from build123d import *

# Parameters (mm, degrees)
SKETCH1_W           = 55
SKETCH1_H           = 28
BOSS_EXTRUDE1_DEPTH = 50
SKETCH2_R           = 14
BOSS_EXTRUDE2_DEPTH = 5
SKETCH3_R           = 3.5
BOSS_EXTRUDE3_DEPTH = 7
SKETCH4_W           = 11
SKETCH4_H           = 28
BOSS_EXTRUDE4_DEPTH = 3
CUT_EXTRUDE1_DEPTH  = 3


with BuildPart() as part:
    # Sketch1 → Boss-Extrude1 (new body)
    with BuildSketch(Plane(origin=(0, 0, 0), x_dir=(1, 0, 0), z_dir=(0, 1, 0))):
        Rectangle(SKETCH1_W, SKETCH1_H)
    extrude(amount=BOSS_EXTRUDE1_DEPTH)

    # Sketch2 → Boss-Extrude2 (add)
    with BuildSketch(Plane(origin=(0, 50, 0), x_dir=(1, 0, 0), z_dir=(0, 1, 0))):
        with Locations(Location((-13.5, 0, 0), (0, 0, 270))):
            Circle(SKETCH2_R)
    extrude(amount=BOSS_EXTRUDE2_DEPTH)

    # Sketch3 → Boss-Extrude3 (add)
    with BuildSketch(Plane(origin=(0, 55, 0), x_dir=(1, 0, 0), z_dir=(0, 1, 0))):
        with Locations(Location((-13.5, 0, 0), (0, 0, 270))):
            Circle(SKETCH3_R)
    extrude(amount=BOSS_EXTRUDE3_DEPTH)

    # Sketch4 → Boss-Extrude4 (add)
    with BuildSketch(Plane(origin=(0, 41.5, 0), x_dir=(1, 0, 0), z_dir=(0, 1, 0))):
        with Locations((33, 0)):
            Rectangle(SKETCH4_W, SKETCH4_H)
        with Locations((-33, 0)):
            Rectangle(SKETCH4_W, SKETCH4_H)
    extrude(amount=BOSS_EXTRUDE4_DEPTH)

    # Sketch5 → Cut-Extrude1 (cut)
    with BuildSketch(Plane(origin=(0, 41.5, 0), x_dir=(1, 0, 0), z_dir=(0, 1, 0))):
        with BuildLine():
            Line((35.949489743, 4.5), (38.5, 4.5))
            Line((38.5, 4.5), (38.5, 9.5))
            Line((38.5, 9.5), (35.949489743, 9.5))
            ThreePointArc((35.949489743, 9.5), (30, 7), (35.949489743, 4.5))
        make_face()
        with BuildLine():
            Line((38.5, -9.5), (38.5, -4.5))
            Line((38.5, -4.5), (35.949489743, -4.5))
            ThreePointArc((35.949489743, -4.5), (30, -7), (35.949489743, -9.5))
            Line((35.949489743, -9.5), (38.5, -9.5))
        make_face()
        with BuildLine():
            Line((-35.949489743, -4.5), (-38.5, -4.5))
            Line((-38.5, -4.5), (-38.5, -9.5))
            Line((-38.5, -9.5), (-35.949489743, -9.5))
            ThreePointArc((-35.949489743, -9.5), (-30, -7), (-35.949489743, -4.5))
        make_face()
        with BuildLine():
            Line((-38.5, 9.5), (-38.5, 4.5))
            Line((-38.5, 4.5), (-35.949489743, 4.5))
            ThreePointArc((-35.949489743, 4.5), (-30, 7), (-35.949489743, 9.5))
            Line((-35.949489743, 9.5), (-38.5, 9.5))
        make_face()
    extrude(amount=CUT_EXTRUDE1_DEPTH, mode=Mode.SUBTRACT)


solid = part.part
Read the model definition and answer for the solid it produces. Units are mm, in the model's axes. A direction names the side the tool comes from. Round coordinates to 2 decimals unless told otherwise and drop trailing zeros. Order: outer loops, then holes, each group sorted by start corner. A loop starts at its lowest first (then second) coordinate and runs counter-clockwise, first axis right, second up.
1) Flat-ended cylindrical pins translate along their axes: pin 1 (14 mm diameter, centred on y = 31, z = -2, fed in from +X); pin 2 (6 mm diameter, centred on x = -17, z = 10, fed in from +Y); pin 3 (9 mm diameter, centred on x = 34, z = -1.5, fed in from +Y). Find the tip coordinate at first contact, or state that the pin passes through.
2) The part is cut by section A-A on x = -33.5. Write down the section's boundary in (y, z), plus the area to 3 significant figures.
3) Straight lines are drawn through the part: L1, parallel to Z at x = 33.5, y = 42.9; L2, parallel to X at y = 11.5, z = 5.25; L3, parallel to Y at x = 19, z = -4.5. For each, find the intervals that lie inside material, in ascending order.
4) The part is cut by section C-C on z = 6.5. Write down the section's boundary in (x, y), plus the area to 3 significant figures.
5) For faces 1 (the face through (-16.605, 58.451, 1.615)), 2 (the face through (27.5, 20, 0)), 3 (the face through (-25, 50, 11)), determine the directions among +Z, -Z, +X, -X, +Y, -Y from which every point of the face is accessible in a straight line to the end or side of a thin tool.
6) The part is cut by section B-B on y = 26. Write down the section's boundary in (x, z).
7) The part is cut by section D-D on x = -3. Write down the section's boundary in (y, z), plus the area to 3 significant figures.
Resolved:
1. pin 1: stops at x = 27.5
1. pin 2: stops at y = 55
1. pin 3: stops at y = 44.5
2. outline: (41.5, -14) - (44.5, -14) - (44.5, -10.5) - (41.5, -10.5) - close; (41.5, -3.5) - (44.5, -3.5) - (44.5, 3.5) - (41.5, 3.5) - close; (41.5, 10.5) - (44.5, 10.5) - (44.5, 14) - (41.5, 14) - close
2. area: 42.0 mm2
3. L1: z = -14 to -10.5, -3.5 to 3.5, 10.5 to 14
3. L2: x = -27.5 to 27.5
3. L3: y = 0 to 50
4. outline: (-30.04, 41.5) - (-27.5, 41.5) - (-27.5, 0) - (27.5, 0) - (27.5, 41.5) - (30.04, 41.5) - (30.04, 44.5) - (27.5, 44.5) - (27.5, 50) - (-1.1, 50) - (-1.1, 55) - (-25.9, 55) - (-25.9, 50) - (-27.5, 50) - (-27.5, 44.5) - (-30.04, 44.5) - close
4. area: 2,890 mm2
5. face 1: +Y
5. face 2: +Z, -Z, +X, -Y
5. face 3: +Z, -X, +Y
6. outline: (-27.5, -14) - (27.5, -14) - (27.5, 14) - (-27.5, 14) - close
7. outline: (0, -14) - (50, -14) - (50, -9.26) - (55, -9.26) - (55, 9.26) - (50, 9.26) - (50, 14) - (0, 14) - close
7. area: 1,490 mm2
